Geometry check sheet. Reference: the model listing, model coordinates, mm. A direction names the side the tool comes from. Give positions to 0.01 mm unless a question says otherwise; leave off trailing zeros. Loops run counter-clockwise (first coordinate to the right, second up) from the corner with the lowest first, then second, coordinate; pieces in that order, holes last. Notation, with made-up numbers: (0.25, 21.25) -> (20.25, 21.25) arc R14 cw to (20.25, 26.25) -> close; hole circle Ø4 at (46.25, 53.25). An arc over 180 degrees is marked (long way). One line per item, written item: value. Start each with the question number.
(1) Sectioned sample at B-B, the plane y = 15. Record the cut outline in (x, z), then the cut area to 3 significant figures.
(2) Tool access check on faces 1 (the face through (0, 38, 10)), 2 (the face through (-1, 23, 21.25)), 3 (the face through (11.25, 11, 0)), 4 (the face through (21.25, 19, 0)), 5 (the face through (-21.25, 20, 0)). Record the directions out of +Z, -Z, +X, -X, +Y, -Y that give a thin tool (end or side, any length) a straight path to the whole face; none if there is none.
(3) Scan lines: line 1 along X through (y, z) = (15.5, 13.5); line 2 along X through (y, z) = (32.75, 0); line 3 along Y through (x, z) = (-4, -1). Record each from-to range of solid material in increasing order. Write a range as from..to.
(4) Draft check along X on faces 6 (the face through (-16.796, 29.479, 0.297)), 7 (the face through (16.95, 29.41, 0.3)), 8 (the face through (0.9, 32.64, 2.86)). Enter one of: pulls with the +X half, pulls with the -X half, needs draft (parallel to the pull), parting line crosses it, or undercut.
(5) Sectioned sample at C-C, the plane z = 0. Record the cut outline in (x, y), then the cut area to 3 significant figures.
(6) Sectioned sample at A-A, the plane x = 0. Record the cut outline in (y, z), then the cut area to 3 significant figures.
(7) Gauge pin test, flat ends, axial feed: pin 1 Ø2.5 at (x, z) = (-29, -6.5) entering from +Y; pin 2 Ø11 at (y, z) = (38.5, -4.5) entering from +X; pin 3 Ø5 at (x, y) = (-3.5, 35.5) entering from -Z. Record the tip position at first contact, or that the pin passes through.
(8) Sectioned sample at D-D, the plane z = -7. Record the cut outline in (x, y), then the cut area to 3 significant figures.
from build123d import *

# Parameters (mm, degrees)
BOSS_EXTRUDE1_DEPTH     = 21.25
CUT_EXTRUDE1_DEPTH      = 60.765165439
CUT_EXTRUDE1_DEPTH_BACK = 60.765165439
SKETCH3_R               = 3
CUT_EXTRUDE2_DEPTH      = 60.765165439


with BuildPart() as part:
    # Sketch1 → Boss-Extrude1 (new, symmetric)
    with BuildSketch(Plane.XY):
        Polygon((-11.25, 0), (-11.25, 22.5), (11.25, 22.5), (11.25, 0), (36.25, 0), (33.25, 5), (25.25, 5), (21.25, 11.666666667), (21.25, 27.5), (10, 32.5), (10, 42.5), (-10, 42.5), (-10, 32.5), (-21.25, 27.5), (-21.25, 11.666666667), (-25.25, 5), (-33.25, 5), (-36.25, 0), align=None)
    extrude(amount=BOSS_EXTRUDE1_DEPTH, both=True)

    # Sketch2 → Cut-Extrude1 (cut, two sides: drawn at the far end of the back side and taken through both)
    with BuildSketch(Plane(origin=(0, 0, 0), x_dir=(0, 0, -1), z_dir=(1, 0, 0)).offset(-CUT_EXTRUDE1_DEPTH_BACK)):
        Polygon((21.25, 27.5), (10, 32.5), (10, 42.5), (21.25, 42.5), align=None)
        Polygon((-10, 42.5), (-10, 32.5), (-21.25, 27.5), (-21.25, 42.5), align=None)
    extrude(amount=CUT_EXTRUDE1_DEPTH + CUT_EXTRUDE1_DEPTH_BACK, mode=Mode.SUBTRACT)

    # Sketch3 → Cut-Extrude2 (cut, through all)
    with BuildSketch(Plane(origin=(0, 42.5, 0), x_dir=(1, 0, 0), z_dir=(0, 1, 0))):
        with Locations(Location((0, 0, 0), (0, 0, 270))):
            Circle(SKETCH3_R)
    extrude(amount=-CUT_EXTRUDE2_DEPTH, mode=Mode.SUBTRACT)


solid = part.part
Calculated:
1. outline: (-21.25, -21.25) -> (-11.25, -21.25) -> (-11.25, 21.25) -> (-21.25, 21.25) -> close; (11.25, -21.25) -> (21.25, -21.25) -> (21.25, 21.25) -> (11.25, 21.25) -> close
1. area: 850 mm2
2. face 1: +Z, +X, -X, +Y
2. face 2: +Z, +X, -X, +Y, -Y
2. face 3: +Z, -Z, -Y
2. face 4: +Z, -Z, +X, +Y
2. face 5: +Z, -Z, -X, +Y
3. line 1: x = -21.25..-11.25, 11.25..21.25
3. line 2: x = -10..-3, 3..10
3. line 3: y = 22.5..42.5
4. face 6: pulls with the -X half
4. face 7: pulls with the +X half
4. face 8: undercut
5. outline: (-36.25, 0) -> (-11.25, 0) -> (-11.25, 22.5) -> (-3, 22.5) -> (-3, 42.5) -> (-10, 42.5) -> (-10, 32.5) -> (-21.25, 27.5) -> (-21.25, 11.67) -> (-25.25, 5) -> (-33.25, 5) -> close; (3, 22.5) -> (11.25, 22.5) -> (11.25, 0) -> (36.25, 0) -> (33.25, 5) -> (25.25, 5) -> (21.25, 11.67) -> (21.25, 27.5) -> (10, 32.5) -> (10, 42.5) -> (3, 42.5) -> close
5. area: 1,060 mm2
6. outline: (22.5, -21.25) -> (27.5, -21.25) -> (32.5, -10) -> (42.5, -10) -> (42.5, -3) -> (22.5, -3) -> close; (22.5, 3) -> (42.5, 3) -> (42.5, 10) -> (32.5, 10) -> (27.5, 21.25) -> (22.5, 21.25) -> close
6. area: 449 mm2
7. pin 1: stops at y = 5
7. pin 2: stops at x = 10
7. pin 3: stops at z = -10
8. outline: (-36.25, 0) -> (-11.25, 0) -> (-11.25, 22.5) -> (11.25, 22.5) -> (11.25, 0) -> (36.25, 0) -> (33.25, 5) -> (25.25, 5) -> (21.25, 11.67) -> (21.25, 27.5) -> (10, 32.5) -> (10, 42.5) -> (-10, 42.5) -> (-10, 32.5) -> (-21.25, 27.5) -> (-21.25, 11.67) -> (-25.25, 5) -> (-33.25, 5) -> close
8. area: 1,180 mm2
